Source: CAD feature listing. Evaluate the final solid. Frame: model axes, mm. Face numbers are marked on the shaded views. Give positions to 0.01 mm unless a question says otherwise; leave off trailing zeros. Loops run counter-clockwise (first coordinate to the right, second up) from the corner with the lowest first, then second, coordinate; pieces in that order, holes last. Notation, with made-up numbers: M 73.5,72.25 L 114.5,72.25 A31 ccw 114.5,98.25 Z; hole C 20,-19 d9. An arc over 180 degrees is marked long. Answer in a Markdown table with one row per item.
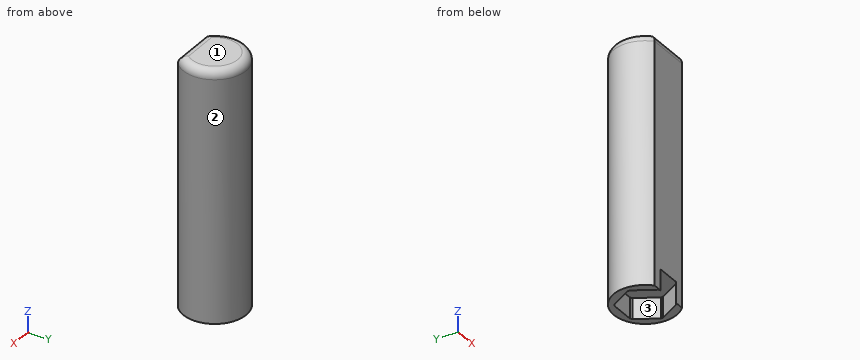
```python
from build123d import *

# Parameters (mm, degrees)
F1_DEPTH    = 30
F2_DEPTH    = 2.5
F3_DEPTH    = 30
F4_T1_DEPTH = 10.1185935568
F4_T4_ANGLE = 350.8041938213


# Not quite as in the source:
# - a fillet or chamfer that OpenCascade refuses, or shapes differently, is made with other operations: its cross-section is extruded or revolved along the edge and cut away or added


with BuildPart() as f1:
    # F0 (on Top) → F1 (new body)
    with BuildSketch(Plane.XY):
        with BuildLine():
            Line((-1.4370107863, -2.775), (-1.602146997, -2.775))
            Line((-1.602146997, -2.775), (-2.5592967784, -2.775))
            ThreePointArc((-2.5592967784, -2.775), (0, -3.775), (2.5592967784, -2.775))
            Line((2.5592967784, -2.775), (1.602146997, -2.775))
            Line((1.602146997, -2.775), (1.4370107863, -2.775))
            ThreePointArc((1.4370107863, -2.775), (0, -3.125), (-1.4370107863, -2.775))
        make_face()
        with BuildLine():
            Line((-1.6847151023, 2.6319878465), (-1.602146997, 2.775))
            Line((-1.602146997, 2.775), (-1.4370107863, 2.775))
            ThreePointArc((-1.4370107863, 2.775), (0, 3.125), (1.4370107863, 2.775))
            Line((1.4370107863, 2.775), (1.602146997, 2.775))
            Line((1.602146997, 2.775), (1.6847151023, 2.6319878465))
            ThreePointArc((1.6847151023, 2.6319878465), (2.7063293868, 1.5625), (3.1217258887, 0.1430121535))
            Line((3.1217258887, 0.1430121535), (3.204293994, 0))
            Line((3.204293994, 0), (3.1217258887, -0.1430121535))
            ThreePointArc((3.1217258887, -0.1430121535), (2.7063293868, -1.5625), (1.6847151023, -2.6319878465))
            Line((1.6847151023, -2.6319878465), (1.602146997, -2.775))
            Line((1.602146997, -2.775), (2.5592967784, -2.775))
            ThreePointArc((2.5592967784, -2.775), (3.4577427853, -1.5148068625), (3.775, 0))
            ThreePointArc((3.775, 0), (-1.5148068625, 3.4577427853), (-2.5592967784, -2.775))
            Line((-2.5592967784, -2.775), (-1.602146997, -2.775))
            Line((-1.602146997, -2.775), (-1.6847151023, -2.6319878465))
            ThreePointArc((-1.6847151023, -2.6319878465), (-2.7063293868, -1.5625), (-3.1217258887, -0.1430121535))
            Line((-3.1217258887, -0.1430121535), (-3.204293994, 0))
            Line((-3.204293994, 0), (-3.1217258887, 0.1430121535))
            ThreePointArc((-3.1217258887, 0.1430121535), (-2.7063293868, 1.5625), (-1.6847151023, 2.6319878465))
        make_face()
        with BuildLine():
            ThreePointArc((3.1217258887, 0.1430121535), (2.7063293868, 1.5625), (1.6847151023, 2.6319878465))
            Line((1.6847151023, 2.6319878465), (3.1217258887, 0.1430121535))
        make_face()
        with BuildLine():
            Line((1.4370107863, -2.775), (-1.4370107863, -2.775))
            ThreePointArc((-1.4370107863, -2.775), (0, -3.125), (1.4370107863, -2.775))
        make_face()
        with BuildLine():
            ThreePointArc((1.4370107863, 2.775), (0, 3.125), (-1.4370107863, 2.775))
            Line((-1.4370107863, 2.775), (1.4370107863, 2.775))
        make_face()
        with BuildLine():
            Line((-3.1217258887, 0.1430121535), (-1.6847151023, 2.6319878465))
            ThreePointArc((-1.6847151023, 2.6319878465), (-2.7063293868, 1.5625), (-3.1217258887, 0.1430121535))
        make_face()
        with BuildLine():
            Line((1.4370107863, 2.775), (-1.4370107863, 2.775))
            ThreePointArc((-1.4370107863, 2.775), (-1.5625, 2.7063293868), (-1.6847151023, 2.6319878465))
            Line((-1.6847151023, 2.6319878465), (-3.1217258887, 0.1430121535))
            ThreePointArc((-3.1217258887, 0.1430121535), (-3.125, 0), (-3.1217258887, -0.1430121535))
            Line((-3.1217258887, -0.1430121535), (-1.6847151023, -2.6319878465))
            ThreePointArc((-1.6847151023, -2.6319878465), (-1.5625, -2.7063293868), (-1.4370107863, -2.775))
            Line((-1.4370107863, -2.775), (1.4370107863, -2.775))
            ThreePointArc((1.4370107863, -2.775), (1.5625, -2.7063293868), (1.6847151023, -2.6319878465))
            Line((1.6847151023, -2.6319878465), (3.1217258887, -0.1430121535))
            ThreePointArc((3.1217258887, -0.1430121535), (3.1241813649, -0.0715248136), (3.125, 0))
            ThreePointArc((3.125, 0), (3.1241813649, 0.0715248136), (3.1217258887, 0.1430121535))
            Line((3.1217258887, 0.1430121535), (1.6847151023, 2.6319878465))
            ThreePointArc((1.6847151023, 2.6319878465), (1.5625, 2.7063293868), (1.4370107863, 2.775))
        make_face()
        with BuildLine():
            Line((-1.6847151023, -2.6319878465), (-3.1217258887, -0.1430121535))
            ThreePointArc((-3.1217258887, -0.1430121535), (-2.7063293868, -1.5625), (-1.6847151023, -2.6319878465))
        make_face()
        with BuildLine():
            ThreePointArc((1.6847151023, -2.6319878465), (2.7063293868, -1.5625), (3.1217258887, -0.1430121535))
            Line((3.1217258887, -0.1430121535), (1.6847151023, -2.6319878465))
        make_face()
        with BuildLine():
            ThreePointArc((-1.4370107863, -2.775), (-1.5625, -2.7063293868), (-1.6847151023, -2.6319878465))
            Line((-1.6847151023, -2.6319878465), (-1.602146997, -2.775))
            Line((-1.602146997, -2.775), (-1.4370107863, -2.775))
        make_face()
        with BuildLine():
            ThreePointArc((1.6847151023, -2.6319878465), (1.5625, -2.7063293868), (1.4370107863, -2.775))
            Line((1.4370107863, -2.775), (1.602146997, -2.775))
            Line((1.602146997, -2.775), (1.6847151023, -2.6319878465))
        make_face()
        with BuildLine():
            Line((3.204293994, 0), (3.1217258887, 0.1430121535))
            ThreePointArc((3.1217258887, 0.1430121535), (3.1241813649, 0.0715248136), (3.125, 0))
            ThreePointArc((3.125, 0), (3.1241813649, -0.0715248136), (3.1217258887, -0.1430121535))
            Line((3.1217258887, -0.1430121535), (3.204293994, 0))
        make_face()
        with BuildLine():
            ThreePointArc((-3.1217258887, -0.1430121535), (-3.125, 0), (-3.1217258887, 0.1430121535))
            Line((-3.1217258887, 0.1430121535), (-3.204293994, 0))
            Line((-3.204293994, 0), (-3.1217258887, -0.1430121535))
        make_face()
        with BuildLine():
            Line((1.602146997, 2.775), (1.4370107863, 2.775))
            ThreePointArc((1.4370107863, 2.775), (1.5625, 2.7063293868), (1.6847151023, 2.6319878465))
            Line((1.6847151023, 2.6319878465), (1.602146997, 2.775))
        make_face()
        with BuildLine():
            Line((-1.4370107863, 2.775), (-1.602146997, 2.775))
            Line((-1.602146997, 2.775), (-1.6847151023, 2.6319878465))
            ThreePointArc((-1.6847151023, 2.6319878465), (-1.5625, 2.7063293868), (-1.4370107863, 2.775))
        make_face()
    extrude(amount=F1_DEPTH)

    # F0 (on Top) → F2 (cut)
    with BuildSketch(Plane.XY):
        with BuildLine():
            Line((1.4370107863, 2.775), (-1.4370107863, 2.775))
            ThreePointArc((-1.4370107863, 2.775), (-1.5625, 2.7063293868), (-1.6847151023, 2.6319878465))
            Line((-1.6847151023, 2.6319878465), (-3.1217258887, 0.1430121535))
            ThreePointArc((-3.1217258887, 0.1430121535), (-3.125, 0), (-3.1217258887, -0.1430121535))
            Line((-3.1217258887, -0.1430121535), (-1.6847151023, -2.6319878465))
            ThreePointArc((-1.6847151023, -2.6319878465), (-1.5625, -2.7063293868), (-1.4370107863, -2.775))
            Line((-1.4370107863, -2.775), (1.4370107863, -2.775))
            ThreePointArc((1.4370107863, -2.775), (1.5625, -2.7063293868), (1.6847151023, -2.6319878465))
            Line((1.6847151023, -2.6319878465), (3.1217258887, -0.1430121535))
            ThreePointArc((3.1217258887, -0.1430121535), (3.1241813649, -0.0715248136), (3.125, 0))
            ThreePointArc((3.125, 0), (3.1241813649, 0.0715248136), (3.1217258887, 0.1430121535))
            Line((3.1217258887, 0.1430121535), (1.6847151023, 2.6319878465))
            ThreePointArc((1.6847151023, 2.6319878465), (1.5625, 2.7063293868), (1.4370107863, 2.775))
        make_face()
    extrude(amount=F2_DEPTH, mode=Mode.SUBTRACT)

    # F0 (on Top) → F3 (cut, through all)
    with BuildSketch(Plane.XY):
        with BuildLine():
            Line((1.4370107863, -2.775), (-1.4370107863, -2.775))
            ThreePointArc((-1.4370107863, -2.775), (0, -3.125), (1.4370107863, -2.775))
        make_face()
        with BuildLine():
            Line((-1.4370107863, -2.775), (-1.602146997, -2.775))
            Line((-1.602146997, -2.775), (-2.5592967784, -2.775))
            ThreePointArc((-2.5592967784, -2.775), (0, -3.775), (2.5592967784, -2.775))
            Line((2.5592967784, -2.775), (1.602146997, -2.775))
            Line((1.602146997, -2.775), (1.4370107863, -2.775))
            ThreePointArc((1.4370107863, -2.775), (0, -3.125), (-1.4370107863, -2.775))
        make_face()
    extrude(amount=F3_DEPTH, mode=Mode.SUBTRACT)

    # F4: fillet of radius 1 on 2 edges, made by hand

    # F4_s2 → F4_t1 (cut)
    with BuildSketch(Plane.YZ.offset(-5.0592967784)):
        with BuildLine():
            ThreePointArc((-2.775, 29), (-2.4821067812, 29.7071067812), (-1.775, 30))
            Line((-1.775, 30), (-2.775, 30))
            Line((-2.775, 30), (-2.775, 29))
        make_face()
    extrude(amount=F4_T1_DEPTH, mode=Mode.SUBTRACT)

    # F4_s3 → F4_t4 (revolve, cut)
    with BuildSketch(Plane(origin=(0, 0, 0), x_dir=(0, 0, 1), z_dir=(-0.9967818129, -0.0801624442, 0))):
        with BuildLine():
            ThreePointArc((29, -3.775), (29.7071067812, -3.4821067812), (30, -2.775))
            Line((30, -2.775), (30, -3.775))
            Line((30, -3.775), (29, -3.775))
        make_face()
    revolve(axis=Axis((0, 0, 30), (0, 0, 1)), revolution_arc=F4_T4_ANGLE, mode=Mode.SUBTRACT)


solid = f1.part
```
1) Section B-B, the plane z = 6.5. Return loops of the section in (x, y) (3 decimals), then the cut area to 3 significant figures.
Reply:
| item | result |
|---|---|
| outline | M -2.559,-2.775 L 2.559,-2.775 A3.775 ccw long Z |
| area | 41.3 mm² |
2) Pin query (flat end, axial travel): pin 1 Ø1.7 at (x, y) = (1, -1) entering from -Z. Return the tip coordinate at first contact, or that it passes through.
Reply:
| item | result |
|---|---|
| pin 1 | stops at z = 2.5 |
3) Material intervals for L1, parallel to Z at x = 0.5, y = 1.5; L2, parallel to X at y = -2.5, z = 5; L3, parallel to Y at x = -3, z = 18, sorted ascending.
Reply:
| item | result |
|---|---|
| L1 | z = 2.5 to 30 |
| L2 | x = -2.83 to 2.83 |
| L3 | y = -2.29 to 2.29 |
4) Pull-direction query (Y, two-part tool) for the marked faces 1, 2 and 3; classes: released by +Y, released by -Y, zero draft, split by the parting line, or undercut.
Reply:
| item | result |
|---|---|
| face 1 | zero draft |
| face 2 | split by the parting line |
| face 3 | undercut |
5) Section A-A, the plane x = 0. Return loops of the section in (y, z) (3 decimals), then the cut area to 3 significant figures.
Reply:
| item | result |
|---|---|
| outline | M -2.775,2.5 L 2.775,2.5 L 2.775,0 L 3.775,0 L 3.775,29 A1 ccw 2.775,30 L -1.775,30 A1 ccw -2.775,29 Z |
| area | 182 mm² |
